Input: part model. Units: mm. Frame: model coordinates. A direction names the side the tool comes from. Give positions to 0.01 mm unless a question says otherwise; leave off trailing zeros. Loops run counter-clockwise (first coordinate to the right, second up) from the corner with the lowest first, then second, coordinate; pieces in that order, holes last.
from build123d import *

# Parameters (mm, degrees)
EXTRUDE_1_DEPTH              = 14
CUT_EXTRUDE_1_DEPTH          = 8.5
SKETCH_3_W                   = 5.5
SKETCH_3_H                   = 7.999
EXTRUDE_2_DEPTH              = 2.4
SKETCH_4_W                   = 5.5
SKETCH_4_H                   = 7.999
EXTRUDE_3_DEPTH              = 2.4
HOLE_WIZARD_12_0_12_1_D      = 12
HOLE_WIZARD_M3_1_D           = 3.2
HOLE_WIZARD_M3_1_CBORE_D     = 6
HOLE_WIZARD_M3_1_CBORE_DEPTH = 4
HOLE_WIZARD_M3_2_D           = 3.2
HOLE_WIZARD_M3_2_DEPTH       = 14
HOLE_WIZARD_M3_2_CBORE_D     = 6
HOLE_WIZARD_M3_2_CBORE_DEPTH = 3.5
FILLET_1_R                   = 0.5
FILLET_2_R                   = 1


with BuildPart() as part:
    # 草图1 → 凸台-拉伸1 (new body)
    with BuildSketch(Plane.XY.offset(14)):
        with BuildLine():
            Line((-7.5, -15.811388301), (-7.5, -48.5))
            Line((-7.5, -48.5), (7.5, -48.5))
            Line((7.5, -48.5), (7.5, -15.811388301))
            ThreePointArc((7.5, -15.811388301), (0, 17.5), (-7.5, -15.811388301))
        make_face()
    extrude(amount=-EXTRUDE_1_DEPTH)

    # 草图2 → 切除-拉伸1 (cut)
    with BuildSketch(Plane(origin=(0, 0, 0), x_dir=(-1, 0, 0), z_dir=(0, 0, -1))):
        with BuildLine():
            Line((7.5, -48.5), (7.5, -18.270536391))
            ThreePointArc((7.5, -18.270536391), (0, -19.75), (-7.5, -18.270536391))
            Line((-7.5, -18.270536391), (-7.5, -48.5))
            Line((-7.5, -48.5), (7.5, -48.5))
        make_face()
    extrude(amount=-CUT_EXTRUDE_1_DEPTH, mode=Mode.SUBTRACT)

    # 草图3 → 凸台-拉伸2 (add)
    with BuildSketch(Plane.ZY.offset(7.5)):
        with Locations((11.25, -44.5005)):
            Rectangle(SKETCH_3_W, SKETCH_3_H)
    extrude(amount=EXTRUDE_2_DEPTH)

    # 草图4 → 凸台-拉伸3 (add)
    with BuildSketch(Plane(origin=(7.5, 0, 0), x_dir=(0, 0, -1), z_dir=(1, 0, 0))):
        with Locations((-11.25, -44.5005)):
            Rectangle(SKETCH_4_W, SKETCH_4_H)
    extrude(amount=EXTRUDE_3_DEPTH)

    # Ø12.0 (12) 直径孔1 (through all)
    with Locations(Plane(origin=(0, 0, 0), x_dir=(-1, 0, 0), z_dir=(0, 0, -1))):
        with Locations((0, 0)):
            Hole(HOLE_WIZARD_12_0_12_1_D / 2)

    # M3 六角头机械螺钉的柱形沉头孔1 (through all)
    with Locations(Plane.XY.offset(14)):
        with Locations((0, 13.5), (11.691342951, 6.75), (11.691342951, -6.75), (0, -13.5), (-11.691342951, -6.75), (-11.691342951, 6.75)):
            CounterBoreHole(HOLE_WIZARD_M3_1_D / 2, HOLE_WIZARD_M3_1_CBORE_D / 2, HOLE_WIZARD_M3_1_CBORE_DEPTH)

    # M3 六角头机械螺钉的柱形沉头孔2
    with Locations(Plane.XY.offset(14)):
        with Locations((0, -38), (5.501, -44.5005), (-5.499, -44.5005)):
            CounterBoreHole(HOLE_WIZARD_M3_2_D / 2, HOLE_WIZARD_M3_2_CBORE_D / 2, HOLE_WIZARD_M3_2_CBORE_DEPTH, depth=HOLE_WIZARD_M3_2_DEPTH)

    # 圆角1
    fillet_1_edges = [part.edges().sort_by_distance(p)[0] for p in [
        (7.5, -18.270536391, 4.25),
        (-7.5, -18.270536391, 4.25),
        (7.5, -15.811388301, 7),
        (-7.5, -15.811388301, 7),
    ]]
    fillet(fillet_1_edges, radius=FILLET_1_R)

    # 圆角2
    fillet_2_edges = [part.edges().sort_by_distance(p)[0] for p in [
        (-7.5, -40.501, 11.25),
        (-9.9, -40.501, 11.25),
        (-9.9, -48.5, 11.25),
        (7.5, -40.501, 11.25),
        (9.9, -40.501, 11.25),
        (9.9, -48.5, 11.25),
    ]]
    fillet(fillet_2_edges, radius=FILLET_2_R)


solid = part.part
(1) Cut plane A-A (y = 0). Return the cut outline in (x, z).
Values follow:
outline: (-17.5, 0) - (-6, 0) - (-6, 14) - (-17.5, 14) - close; (6, 0) - (17.5, 0) - (17.5, 14) - (6, 14) - close
(2) Cut plane D-D (x = -5). Return the cut outline in (y, z), and give its area (3 significant figures).
Values follow:
outline: (-48.5, 8.5) - (-46.02, 8.5) - (-46.02, 10.5) - (-47.46, 10.5) - (-47.46, 14) - (-48.5, 14) - close; (-42.98, 8.5) - (-19.11, 8.5) - (-19.11, 0) - (-3.32, 0) - (-3.32, 14) - (-41.54, 14) - (-41.54, 10.5) - (-42.98, 10.5) - close; (3.32, 0) - (16.77, 0) - (16.77, 14) - (3.32, 14) - close
area: 544 mm2
(3) Mould query, pull axis Y, two halves, no side actions, for faces 1 (the flat face through (-10, 5, 10)), 2 (the flat face through (4, -5, 0)), 3 (the cylindrical face through (-0.1, -19.75, 4.19)). Classes: +Y half, -Y half, draft (parallel to the pull), parting line (faces both ways), or undercut.
Values follow:
face 1: undercut
face 2: draft
face 3: -Y half
(4) Cut plane C-C (z = 7.25). Return the cut outline in (x, y).
Values follow:
outline: (-7.78, -15.68) arc R0.5 cw to (-7.5, -16.12) - (-7.5, -17.93) arc R0.5 ccw to (-7.18, -18.4) arc R19.75 ccw to (7.18, -18.4) arc R0.5 ccw to (7.5, -17.93) - (7.5, -16.12) arc R0.5 cw to (7.78, -15.68) arc R17.5 ccw (long way) to start; hole circle Ø3.2 at (-11.69, -6.75); hole circle Ø3.2 at (-11.69, 6.75); hole circle Ø12 at (0, 0); hole circle Ø3.2 at (0, -13.5); hole circle Ø3.2 at (0, 13.5); hole circle Ø3.2 at (11.69, -6.75); hole circle Ø3.2 at (11.69, 6.75)
(5) Cut plane B-B (x = 0). Count the separate pieces of the cut face and the enclosed holes in it, and give its area (3 significant figures).
Values follow:
separate pieces: 5
enclosed holes: 0
area: 372 mm2
(6) Reachability of faces 4 (the cylindrical face through (-0.74, -39.42, 9.49)), 5 (the flat face through (1, -15, 10)), 6 (the flat face through (7.5, -28, 10)) from +Z, -Z, +X, -X, +Y, -Y: full face, straight path, thin tool, end or side. Return the list, or none.
Values follow:
face 4: +Z, -Z
face 5: +Z
face 6: +Z, -Z, +X
(7) Pin query (flat end, axial travel): pin 1 Ø1.5 at (x, z) = (-11, 3.5) entering from +Y; pin 2 Ø4 at (x, y) = (1.5, -34) entering from -Z; pin 3 Ø4 at (x, y) = (-5.5, -44.5) entering from +Z; pin 4 Ø9.5 at (x, y) = (-11.69, 6.75) entering from -Z. Return the tip coordinate at first contact, or that it passes through.
Values follow:
pin 1: stops at y = 14.18
pin 2: stops at z = 8.5
pin 3: stops at z = 10.5
pin 4: stops at z = 0
(8) Ray query, probe 1 along Y at (x, z) = (0, 3); probe 2 along Y at (x, z) = (1, 12); probe 3 along X at (y, z) = (9, 13.25). Return the intervals inside material, ascending.
Values follow:
probe 1: y = -19.75 to -15.1, -11.9 to -6, 6 to 11.9, 15.1 to 17.5
probe 2: y = -48.5 to -40.83, -35.17 to -16.33, -10.67 to -5.92, 5.92 to 10.67, 16.33 to 17.47
probe 3: x = -15.01 to -13.68, -9.71 to 9.71, 13.68 to 15.01
